Could you check a few things on this model? Use its own coordinates, in mm. Face numbers are marked on the shaded views. A direction names the side the tool comes from. Coordinates: 2 decimals unless noted, no trailing zeros. Write each loop counter-clockwise with the first axis right and the second up, starting at its lowest first coordinate (ties: lowest second). Pieces come first, ordered by that corner, then holes. Notation, with made-up numbers: M -28,38.5 L 28,38.5 A24 ccw 28,77.5 Z; hole C 79,15 d4. An arc over 180 degrees is marked long. Write item = value, one per line.
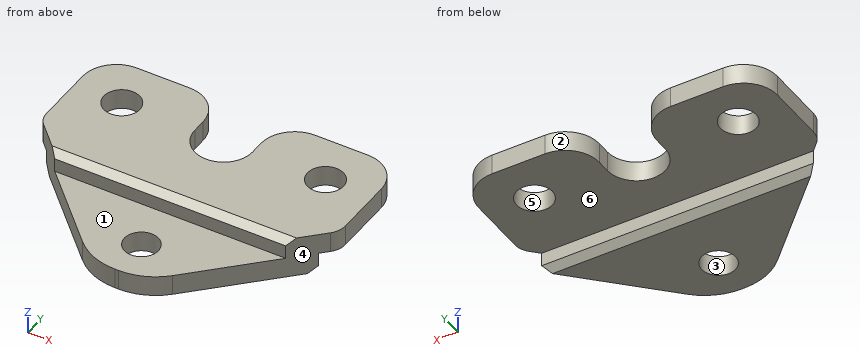
```python
from build123d import *

# Parameters (mm, degrees)
SKETCH_R        = 2.65
PAD_DEPTH       = 3
PAD001_DEPTH    = 3
SKETCH002_R     = 2.5
PAD002_DEPTH    = 3
FILLET_R        = 9
FILLET001_R     = 5
FILLET002_R     = 5
CHAMFER_SIZE    = 1
CHAMFER001_SIZE = 1
FILLET003_R     = 3


with BuildPart() as part:
    # Sketch → Pad (new body)
    with BuildSketch(Plane.XY):
        with BuildLine():
            ThreePointArc((-4.25, 0), (0, -4.25), (4.25, 0))
            Line((4.25, 7), (4.25, 0))
            Line((22, 7), (4.25, 7))
            Line((22, -8), (22, 7))
            Line((22, -8), (17, -13))
            Line((-17, -13), (17, -13))
            Line((-22, -8), (-17, -13))
            Line((-22, 7), (-22, -8))
            Line((-4.25, 7), (-22, 7))
            Line((-4.25, 0), (-4.25, 7))
        make_face()
        with Locations((-15, 0)):
            Circle(SKETCH_R, mode=Mode.SUBTRACT)
        with Locations((15, 0)):
            Circle(SKETCH_R, mode=Mode.SUBTRACT)
    extrude(amount=PAD_DEPTH)

    # Sketch001 → Pad001 (join)
    with BuildSketch(Plane.XY):
        Polygon((-17, -13), (17, -13), (20, -10), (-20, -10), align=None)
    extrude(amount=-PAD001_DEPTH)

    # Sketch002 → Pad002 (join)
    with BuildSketch(Plane.XY):
        Polygon((-17, -13), (17, -13), (4, -26), (-4, -26), align=None)
        with Locations((0, -20)):
            Circle(SKETCH002_R, mode=Mode.SUBTRACT)
    extrude(amount=-PAD002_DEPTH)

    # Fillet
    fillet_edges = [part.edges().sort_by_distance(p)[0] for p in [
        (4, -26, -1.5),
        (-4, -26, -1.5),
    ]]
    fillet(fillet_edges, radius=FILLET_R)

    # Fillet001
    fillet001_edges = [part.edges().sort_by_distance(p)[0] for p in [
        (22, 7, 1.5),
        (-22, 7, 1.5),
    ]]
    fillet(fillet001_edges, radius=FILLET001_R)

    # Fillet002
    fillet002_edges = [part.edges().sort_by_distance(p)[0] for p in [
        (-4.25, 7, 1.5),
        (4.25, 7, 1.5),
    ]]
    fillet(fillet002_edges, radius=FILLET002_R)

    # Chamfer
    chamfer_edges = [part.edges().sort_by_distance(p)[0] for p in [
        (0, -13, 3),
    ]]
    chamfer(chamfer_edges, length=CHAMFER_SIZE)

    # Chamfer001
    chamfer001_edges = [part.edges().sort_by_distance(p)[0] for p in [
        (0, -10, -3),
    ]]
    chamfer(chamfer001_edges, length=CHAMFER001_SIZE)

    # Fillet003
    fillet003_edges = [part.edges().sort_by_distance(p)[0] for p in [
        (22, -8, 1.5),
        (-22, -8, 1.5),
    ]]
    fillet(fillet003_edges, radius=FILLET003_R)


solid = part.part
```
Item 1: If I drill on line 1 along Y through (x, z) = (15, 1.55); line 2 along Y through (x, z) = (0, -0.8); line 3 along Z through (x, y) = (-6, -22), over which ranges is the centre line in solid material (lowest first)?
Numbers:
line_1 = -13 to -2.65, 2.65 to 7
line_2 = -26 to -22.5, -17.5 to -10
line_3 = -3 to 0
Item 2: I'm going to push flat-ended pins straight in: P1, Ø1.5, axis at x = -3.5, z = -1, coming from the +Y side; P2, Ø10.5, axis at x = -2, y = -22, coming from the +Z side; P3, Ø7, axis at x = -15, y = 0, coming from the -Z side. Where does each tip first touch, or does it pass through?
Numbers:
P1 = -10
P2 = 0
P3 = 0
Item 3: For the marked faces 1, 2 and 3, which set-ups out of +Z, -Z, +X, -X, +Y, -Y let a thin tool reach every point of the face, with its end or its side?
Numbers:
face_1 = +Z, +X, -X, -Y
face_2 = +Z, -Z, +Y
face_3 = +Z, -Z
Item 4: If we mould it in two halves opening along X, with no side actions, what happens to the marked faces 4, 5 and 6? For each: pulls with the +X half, pulls with the -X half, needs draft (parallel to the pull), parting line crosses it, or undercut.
Numbers:
face_4 = pulls with the +X half
face_5 = undercut
face_6 = needs draft
Item 5: Imagine slicing it at B-B (y = -20). Write out the boundary of the cut face in (x, z).
Numbers:
outline = M -10,-3 L -2.5,-3 L -2.5,0 L -10,0 Z; M 2.5,-3 L 10,-3 L 10,0 L 2.5,0 Z
Item 6: Imagine slicing it at A-A (x = 15). Write out the boundary of the cut face in (y, z).
Numbers:
outline = M -15,-3 L -11,-3 L -10,-2 L -10,0 L -2.65,0 L -2.65,3 L -12,3 L -13,2 L -13,0 L -15,0 Z; M 2.65,0 L 7,0 L 7,3 L 2.65,3 Z
Item 7: Imagine slicing it at D-D (x = -1). Write out the boundary of the cut face in (y, z), and give its area (3 significant figures).
Numbers:
outline = M -25.97,-3 L -22.29,-3 L -22.29,0 L -25.97,0 Z; M -17.71,-3 L -11,-3 L -10,-2 L -10,0 L -4.13,0 L -4.13,3 L -12,3 L -13,2 L -13,0 L -17.71,0 Z
area = 59.8 mm²
Item 8: Imagine slicing it at C-C (z = 1). Write out the boundary of the cut face in (x, y).
Numbers:
outline = M -22,-6.76 A3 ccw -21.12,-8.88 L -17,-13 L 17,-13 L 21.12,-8.88 A3 ccw 22,-6.76 L 22,2 A5 ccw 17,7 L 9.25,7 A5 ccw 4.25,2 L 4.25,0 A4.25 cw -4.25,0 L -4.25,2 A5 ccw -9.25,7 L -17,7 A5 ccw -22,2 Z; hole C -15,0 d5.3; hole C 15,0 d5.3
